```python
from build123d import *

# Parameters (mm, degrees)
SKETCH1_W                                           = 30
SKETCH1_H                                           = 60
BOSS_EXTRUDE1_DEPTH                                 = 6
CUT_EXTRUDE1_DEPTH                                  = 3
CUT_EXTRUDE2_DEPTH                                  = 34.674916481
FILLET1_R                                           = 3
CHAMFER1_SIZE                                       = 1.5
CBORE_FOR_M6_HEX_SOCKET_HEAD_CAP_SCREW1_D           = 6.6
CBORE_FOR_M6_HEX_SOCKET_HEAD_CAP_SCREW1_CBORE_D     = 11
CBORE_FOR_M6_HEX_SOCKET_HEAD_CAP_SCREW1_CBORE_DEPTH = 2


with BuildPart() as part:
    # Sketch1 → Boss-Extrude1 (new body)
    with BuildSketch(Plane(origin=(0, 0, 0), x_dir=(1, 0, 0), z_dir=(0, 1, 0))):
        Rectangle(SKETCH1_W, SKETCH1_H)
    extrude(amount=BOSS_EXTRUDE1_DEPTH)

    # Sketch2 → Cut-Extrude1 (cut)
    with BuildSketch(Plane.XZ):
        Polygon((15, -6), (-9, -30), (15, -30), align=None)
    extrude(amount=-CUT_EXTRUDE1_DEPTH, mode=Mode.SUBTRACT)

    # Sketch3 → Cut-Extrude2 (cut, through all)
    with BuildSketch(Plane.XZ.offset(-3)):
        Polygon((15, -23.282485579), (15, -30), (8.282485579, -30), align=None)
    extrude(amount=-CUT_EXTRUDE2_DEPTH, mode=Mode.SUBTRACT)

    # Fillet1
    fillet1_edges = [part.edges().sort_by_distance(p)[0] for p in [
        (15, 1.5, -6),
        (-9, 1.5, -30),
        (8.282485579, 4.5, -30),
        (15, 4.5, -23.282485579),
        (15, 3, 30),
        (-15, 3, 30),
        (-15, 3, -30),
    ]]
    fillet(fillet1_edges, radius=FILLET1_R)

    # Chamfer1
    chamfer1_edges = [part.edges().sort_by_distance(p)[0] for p in [
        (15, 6, 2.480077554),
        (-2.480077554, 6, -30),
        (0, 6, 30),
        (-15, 6, 0),
        (11.641242789, 6, -26.641242789),
        (14.121320344, 6, 29.121320344),
        (14.771638598, 6, -23.187895189),
        (8.187895189, 6, -29.771638598),
        (-14.121320344, 6, -29.121320344),
        (-14.121320344, 6, 29.121320344),
    ]]
    chamfer(chamfer1_edges, length=CHAMFER1_SIZE)

    # CBORE for M6 Hex Socket Head Cap Screw1 (through all)
    with Locations(Plane(origin=(0, 6, 0), x_dir=(1, 0, 0), z_dir=(0, 1, 0))):
        with Locations((0, -15), (0, 15)):
            CounterBoreHole(CBORE_FOR_M6_HEX_SOCKET_HEAD_CAP_SCREW1_D / 2, CBORE_FOR_M6_HEX_SOCKET_HEAD_CAP_SCREW1_CBORE_D / 2, CBORE_FOR_M6_HEX_SOCKET_HEAD_CAP_SCREW1_CBORE_DEPTH)


solid = part.part
```
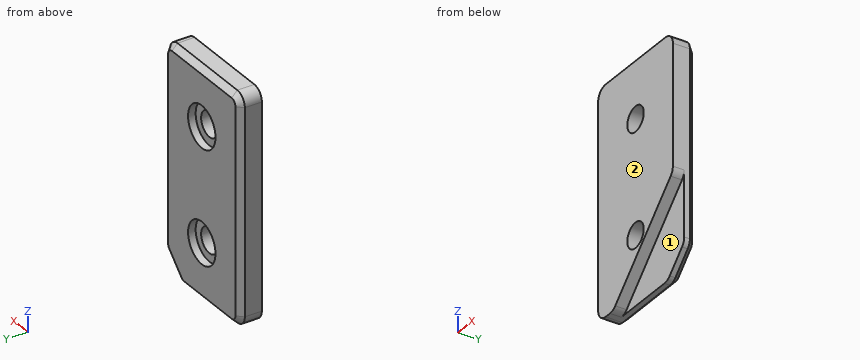
Here's how the part is built. I have some questions about the finished solid (model axes, mm). Face numbers are marked on the shaded views. A direction names the side the tool comes from. Round coordinates to 2 decimals unless told otherwise and drop trailing zeros. Write each loop counter-clockwise with the first axis right and the second up, starting at its lowest first coordinate (ties: lowest second). Pieces come first, ordered by that corner, then holes. Notation, with made-up numbers: M 66,14 L 125,14 A13 cw 125,20 Z; hole C 20.25,-16 d10. An arc over 180 degrees is marked long. Answer as CSV lines item,"result". Start each with the question number.
1. I need wall thicknesses on probe 1 along X at (y, z) = (2.05, -15); probe 2 along Z at (x, y) = (-0.5, 4.5); probe 3 along Z at (x, y) = (1, 1). Which ranges of each line are inside material? Lowest first, please.
2. Suppose I cut it at C-C on x = -7.25. Write out the boundary of the cut face in (y, z), then the cut area to 4 significant figures.
3. On a 3-axis mill with a long thin cutter (end or side, diameter ignored), from which of +Z, -Z, +X, -X, +Y, -Y can I reach the whole of each face in a straight line? I mean the marked faces 1 and 2. Say none if no direction works.
4. I'm going to push flat-ended pins straight in: pin 1 Ø8.5 at (x, z) = (0, -15) entering from +Y; pin 2 Ø10 at (x, z) = (-4.5, 13.5) entering from +Y. Where does each tip first touch, or does it pass through?
5. Suppose I cut it at D-D on z = -15. Write out the boundary of the cut face in (x, y), then the cut area to 3 significant figures.
6. Suppose I cut it at A-A on x = 0. Write out the boundary of the cut face in (y, z).
7. Suppose I cut it at B-B on z = 15. Write out the boundary of the cut face in (x, y), then the cut area to 3 significant figures.
Check result:
1,probe 1,"x = -15 to -3.3, 3.3 to 6"
1,probe 2,"z = -30 to -20.48, -9.52 to 9.52, 20.48 to 30"
1,probe 3,"z = -20 to -18.14, -11.86 to 11.86, 18.14 to 30"
2,outline,"M 0,-28.25 L 3,-28.25 L 3,-30 L 4.5,-30 L 6,-28.5 L 6,28.5 L 4.5,30 L 0,30 Z"
2,area,"352.5 mm2"
3,face 1,"-Z, +X, -Y"
3,face 2,"+Z, -Z, +X, -X, -Y"
4,pin 1,"stops at y = 4"
4,pin 2,"stops at y = 6"
5,outline,"M -15,0 L -3.3,0 L -3.3,4 L -5.5,4 L -5.5,6 L -13.5,6 L -15,4.5 Z; M 3.3,0 L 6,0 L 6,3 L 15,3 L 15,4.5 L 13.5,6 L 5.5,6 L 5.5,4 L 3.3,4 Z"
5,area,"102 mm2"
6,outline,"M 0,-21 L 3,-21 L 3,-30 L 4.5,-30 L 6,-28.5 L 6,-20.5 L 4,-20.5 L 4,-18.3 L 0,-18.3 Z; M 0,-11.7 L 4,-11.7 L 4,-9.5 L 6,-9.5 L 6,9.5 L 4,9.5 L 4,11.7 L 0,11.7 Z; M 0,18.3 L 4,18.3 L 4,20.5 L 6,20.5 L 6,28.5 L 4.5,30 L 0,30 Z"
7,outline,"M -15,0 L -3.3,0 L -3.3,4 L -5.5,4 L -5.5,6 L -13.5,6 L -15,4.5 Z; M 3.3,0 L 15,0 L 15,4.5 L 13.5,6 L 5.5,6 L 5.5,4 L 3.3,4 Z"
7,area,"129 mm2"
